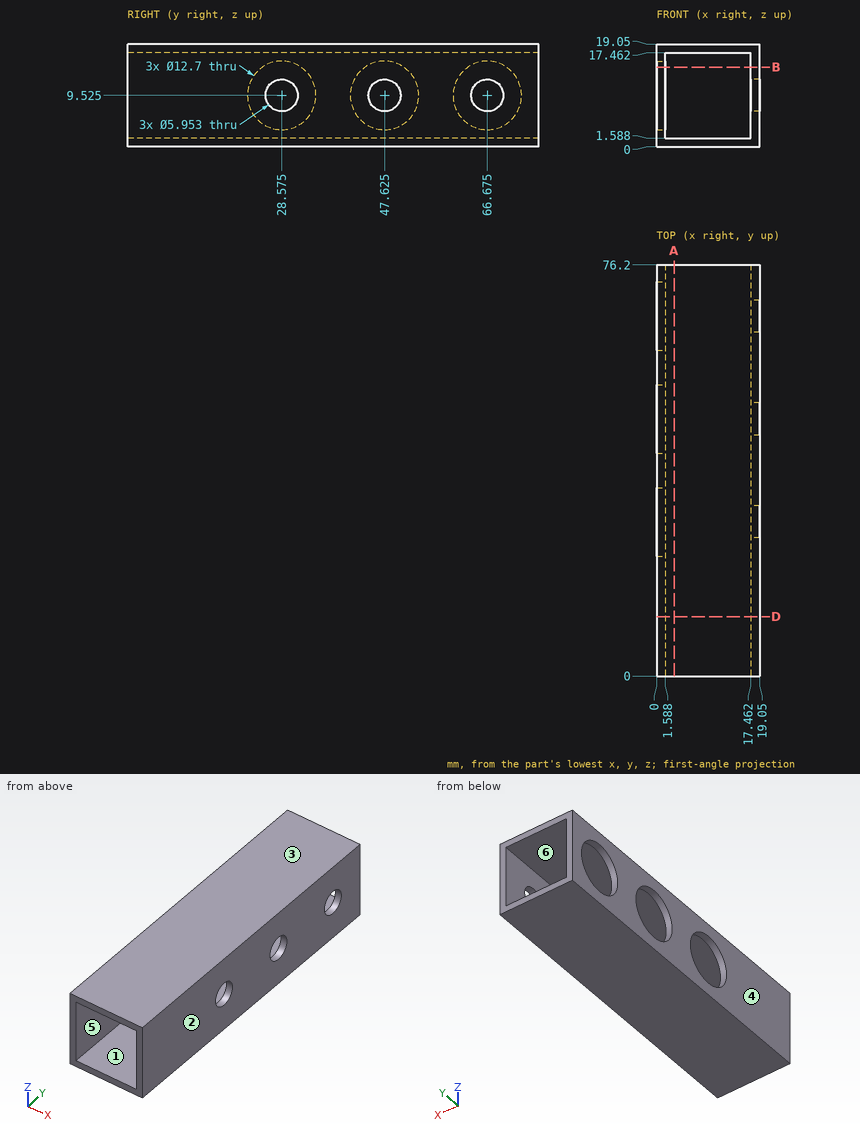
Verification items for this drawing (mm, ordinates from the low corner). A direction names the side the tool comes from. Give positions to 0.01 mm unless a question says otherwise; leave off trailing zeros. Loops run counter-clockwise (first coordinate to the right, second up) from the corner with the lowest first, then second, coordinate; pieces in that order, holes last.
1. Cross-section at A-A on x = 3.25. Record the cut outline in (y, z), and give its area (3 significant figures).
Derived:
outline: (0, 0) - (76.2, 0) - (76.2, 1.59) - (0, 1.59) - close; (0, 17.46) - (76.2, 17.46) - (76.2, 19.05) - (0, 19.05) - close
area: 242 mm2
2. Cross-section at D-D on y = 11. Record the cut outline in (x, z).
Derived:
outline: (0, 0) - (19.05, 0) - (19.05, 19.05) - (0, 19.05) - close; hole (1.59, 1.59) - (17.46, 1.59) - (17.46, 17.46) - (1.59, 17.46) - close
3. Go/stop test with flat-tipped pins: P1, Ø7.5, axis at y = 28.575, z = 9.525, coming from the +X side; P2, Ø7, axis at y = 47.625, z = 9.525, coming from the -X side. Record where each tip stops, or that it passes through.
Derived:
P1: stops at x = 19.05
P2: stops at x = 17.46
4. Material ranges on probe 1 along Z at (x, y) = (12, 73); probe 2 along X at (y, z) = (64, 14.5), recorded low to high.
Derived:
probe 1: z = 0 to 1.59, 17.46 to 19.05
probe 2: x = 17.46 to 19.05
5. Release check for a two-part mould opening along X. For the marked faces 3, 4, 5 and 6 record: +X half, -X half, draft (parallel to the pull), parting line (faces both ways), or undercut.
Derived:
face 3: draft
face 4: -X half
face 5: undercut
face 6: undercut
6. Tool access check on the marked faces 1 and 2. Record the directions out of +Z, -Z, +X, -X, +Y, -Y that give a thin tool (end or side, any length) a straight path to the whole face; none if there is none.
Derived:
face 1: +Y, -Y
face 2: +Z, -Z, +X, +Y, -Y
7. Cross-section at B-B on z = 14.75. Record the cut outline in (x, y).
Derived:
outline: (0, 0) - (1.59, 0) - (1.59, 24.97) - (0, 24.97) - close; (0, 32.18) - (1.59, 32.18) - (1.59, 44.02) - (0, 44.02) - close; (0, 51.23) - (1.59, 51.23) - (1.59, 63.07) - (0, 63.07) - close; (0, 70.28) - (1.59, 70.28) - (1.59, 76.2) - (0, 76.2) - close; (17.46, 0) - (19.05, 0) - (19.05, 76.2) - (17.46, 76.2) - close
